Verification items for the finished model (mm, model axes). Face numbers are marked on the shaded views. Round coordinates to 2 decimals unless told otherwise and drop trailing zeros. Write each loop counter-clockwise with the first axis right and the second up, starting at its lowest first coordinate (ties: lowest second). Pieces come first, ordered by that corner, then holes. Notation, with made-up numbers: (-22, 27) - (0, 27) arc R14 cw to (0, 33) - close; hole circle Ø5 at (10.5, 60.25). An arc over 180 degrees is marked (long way). Answer as a JSON object with one key per item and string values. Group by question number.
1) Section check B-B (y = -1). Enter the section's corners in (x, z).
2) Section check A-A (z = 5). Enter the section's corners in (x, y).
3) Section check D-D (x = 27). Enter the section's corners in (y, z).
4) Thickness scan on line 1 (X direction, y = -10.75, z = 8.5); line 2 (Y direction, x = 26, z = 1.5); line 3 (X direction, y = -9, z = 0.75). Record the ranges inside material, lowest first.
5) Go/stop test with flat-tipped pins: pin 1 Ø2.5 at (x, y) = (-13.92, -10.81) entering from +Z; pin 2 Ø10.5 at (x, y) = (6.08, -5.81) entering from +Z. Record where each tip stops, or that it passes through.
6) Mould release check, pull along Z, two halves, no side actions. Record for the marked faces 1, 2, 3 and 4: +Z half, -Z half, draft (parallel to the pull), parting line (faces both ways), or undercut.
7) Section check C-C (y = -7.25). Enter the section's corners in (x, z), then the cut area to 3 significant figures.
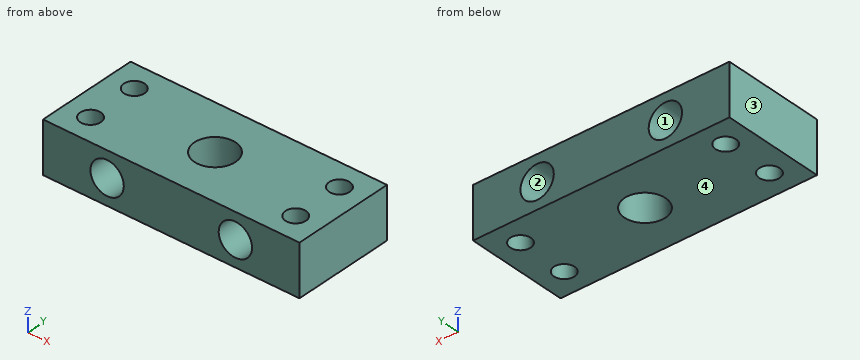
Autodesk Inventor part; units mm, degrees
ref_plane "YZ Plane" through (0, 0, 0) normal (1, 0, 0) x (0, 1, 0)
ref_plane "XZ Plane" through (0, 0, 0) normal (0, 1, 0) x (-1, 0, 0)
ref_plane "XY Plane" through (0, 0, 0) normal (0, 0, 1) x (1, 0, 0)
sketch "Sketch1" plane through (0, 0, 0) normal (0, 0, 1) x (1, 0, 0)
  line L0 (-18.9222, 4.1916) -> (31.0778, 4.1916)
  line L1 (31.0778, 4.1916) -> (31.0778, -15.8084)
  line L2 (31.0778, -15.8084) -> (-18.9222, -15.8084)
  line L3 (-18.9222, -15.8084) -> (-18.9222, 4.1916)
  dimension "d2" = 50
  dimension "d3" = 20
extrude "Extrusion1" add sketch "Sketch1" along normal blind 10
sketch "Sketch2" plane through (-18.9222, -15.8084, 0) normal (0, -1, 0) x (1, 0, 0)
  line L0 (0, 0) -> (0, 10)
  line L1 (50, 0) -> (50, 10)
  point P0 (18.9222, 0)
  point P1 (12.5, 5)
  point P2 (37.5, 5)
  dimension "d6" = 12.5
  dimension "d7" = 12.5
  dimension "d35" = 50
hole "Hole1" at (-6.4222, -15.8084, 5) at (18.5778, -15.8084, 5) direction (0, 1, 0) diameter 6.5 end through all
sketch "Sketch3" plane through (0, 0, 10) normal (0, 0, 1) x (1, 0, 0)
  line L0 (31.0778, 4.1916) -> (31.0778, -15.8084)
  line L1 (31.0778, -15.8084) -> (-18.9222, -15.8084)
  point P0 (0, 0)
  point P1 (6.0778, -5.8084)
  dimension "d36" = 20
  dimension "d37" = 50
  dimension "d38" = 25
  dimension "d39" = 10
hole "Hole2" at (6.0778, -5.8084, 10) direction (0, 0, -1) diameter 8 end through all
sketch "Sketch4" plane through (0, 0, 10) normal (0, 0, 1) x (1, 0, 0)
  line L0 (-18.9222, -15.8084) -> (-18.9222, 4.1916)
  line L1 (31.0778, -15.8084) -> (-18.9222, -15.8084)
  line L2 (-13.9222, -0.8084) -> (26.0778, -0.8084)
  line L3 (26.0778, -0.8084) -> (26.0778, -10.8084)
  line L4 (26.0778, -10.8084) -> (-13.9222, -10.8084)
  line L5 (-13.9222, -10.8084) -> (-13.9222, -0.8084)
  point P0 (31.0778, 4.1916)
  point P1 (0, 0)
  dimension "d22" = 50
  dimension "d23" = 40
  dimension "d24" = 10
  dimension "d25" = 20
  dimension "d26" = 5
  dimension "d27" = 5
hole "Hole3" at (-13.9222, -0.8084, 10) at (26.0778, -0.8084, 10) at (26.0778, -10.8084, 10) at (-13.9222, -10.8084, 10) direction (0, 0, -1) diameter 4 end through all
equation "\"d26\" = -0.5 * d24 + 0.5 * d25"
equation "\"d27\" = -0.5 * d23 + 0.5 * d22"
properties part number "montura tensor"
Returned:
{
 "1": {"outline": "(-18.92, 0) - (-15.91, 0) - (-15.91, 10) - (-18.92, 10) - close; (-11.93, 0) - (24.09, 0) - (24.09, 10) - (-11.93, 10) - close; (28.07, 0) - (31.08, 0) - (31.08, 10) - (28.07, 10) - close; hole circle Ø6.5 at (-6.42, 5); hole circle Ø6.5 at (18.58, 5)"},
 "2": {"outline": "(-18.92, -15.81) - (-9.67, -15.81) - (-9.67, 4.19) - (-18.92, 4.19) - close; (-3.17, -15.81) - (15.33, -15.81) - (15.33, 4.19) - (-3.17, 4.19) - close; (21.83, -15.81) - (31.08, -15.81) - (31.08, 4.19) - (21.83, 4.19) - close; hole circle Ø4 at (-13.92, -10.81); hole circle Ø4 at (-13.92, -0.81); hole circle Ø8 at (6.08, -5.81); hole circle Ø4 at (26.08, -10.81); hole circle Ø4 at (26.08, -0.81)"},
 "3": {"outline": "(-15.81, 0) - (-12.58, 0) - (-12.58, 10) - (-15.81, 10) - close; (-9.03, 0) - (-2.58, 0) - (-2.58, 10) - (-9.03, 10) - close; (0.97, 0) - (4.19, 0) - (4.19, 10) - (0.97, 10) - close"},
 "4": {"line 1": "-18.92 to -15.92, -11.92 to 24.08, 28.08 to 31.08", "line 2": "-15.81 to -12.81, -8.81 to -2.81, 1.19 to 4.19", "line 3": "-18.92 to -14.78, -13.07 to 3.67, 8.49 to 25.22, 26.93 to 31.08"},
 "5": {"pin 1": "through", "pin 2": "z = 10"},
 "6": {"face 1": "undercut", "face 2": "undercut", "face 3": "draft", "face 4": "-Z half"},
 "7": {"outline": "(-18.92, 0) - (2.35, 0) - (2.35, 10) - (-18.92, 10) - close; (9.81, 0) - (31.08, 0) - (31.08, 10) - (9.81, 10) - close; hole circle Ø6.5 at (-6.42, 5); hole circle Ø6.5 at (18.58, 5)", "area": "359 mm2"}
}
